from build123d import *

# Parameters (mm, degrees)
F0_R     = 50
F1_DEPTH = 10
F2_T     = -2.5
F3_W     = 4.3
F3_H     = 4.3
F4_DEPTH = 25


with BuildPart() as f1:
    # F0 (on Top) → F1 (new body)
    with BuildSketch(Plane.XY):
        with Locations((-0.804745, 0.344891)):
            Circle(F0_R)
    extrude(amount=F1_DEPTH)

    # F2
    f2_openings = [f1.faces().sort_by_distance(p)[0] for p in [
        (-0.804745, 0.344891, 10),
    ]]
    offset(amount=F2_T, openings=f2_openings)

    # F3 (on Top) → F4 (join)
    with BuildSketch(Plane.XY):
        with Locations((47.132396, -0.684507)):
            Rectangle(F3_W, F3_H)
    extrude(amount=F4_DEPTH)


solid = f1.part
Geometry check sheet. Reference: the model listing, model coordinates, mm. A direction names the side the tool comes from. Coordinates: 2 decimals unless noted, no trailing zeros. Order: outer loops, then holes, each group sorted by start corner. A loop starts at its lowest first (then second) coordinate and runs counter-clockwise, first axis right, second up. Notation, with made-up numbers: M 60.25,40.25 L 69.25,40.25 A7 ccw 69.25,52.25 Z; hole C 16,52 d6. An arc over 180 degrees is marked long. Use CSV: the item, a comma, the result in double quotes.
Item 1: Mould release check, pull along Y, two halves, no side actions. Record for faces 1 (the flat face through (47, -2.835, 15)), 2 (the flat face through (-1, 1, 2.5)), 3 (the cylindrical face through (-50.702, 3.542, 4.93)), 4 (the flat face through (47, -1, 25)): pulls with the +Y half, pulls with the -Y half, needs draft (parallel to the pull), parting line crosses it, or undercut.
Returned:
face 1,"undercut"
face 2,"undercut"
face 3,"parting line crosses it"
face 4,"needs draft"
Item 2: Gauge pin test, flat ends, axial feed: pin 1 Ø12 at (y, z) = (-22.5, 11.5) entering from +X; pin 2 Ø1 at (x, y) = (-37.5, -27) entering from +Z; pin 3 Ø6 at (y, z) = (7, 10.5) entering from +X. Record the tip position at first contact, or that the pin passes through.
Returned:
pin 1,"stops at x = 46.2"
pin 2,"stops at z = 2.5"
pin 3,"stops at x = 49.06"
Item 3: Cross-section at C-C on x = 23. Record the cut outline in (y, z), then the cut area to 3 significant figures.
Returned:
outline,"M -43.62,0 L 44.31,0 L 44.31,10 L 41.45,10 L 41.45,2.5 L -40.76,2.5 L -40.76,10 L -43.62,10 Z"
area,"263 mm2"
Item 4: Tool access check on faces 5 (the flat face through (49.282, -1, 12)), 6 (the flat face through (44.982, -1, 14)). Record the directions out of +Z, -Z, +X, -X, +Y, -Y that give a thin tool (end or side, any length) a straight path to the whole face; none if there is none.
Returned:
face 5,"+Z, -Z, +X, +Y, -Y"
face 6,"+Z"
Item 5: Thickness scan on line 1 along X through (y, z) = (-0.5, 4.5); line 2 along Z through (x, y) = (-25.5, -8.5); line 3 along X through (y, z) = (-34, 4.5). Record the ranges inside material, lowest first.
Returned:
line 1,"x = -50.8 to -48.3, 44.98 to 49.28"
line 2,"z = 0 to 2.5"
line 3,"x = -37.14 to -33.62, 32.01 to 35.53"
Item 6: Cross-section at D-D on z = 23. Record the cut outline in (x, y), then the cut area to 3 significant figures.
Returned:
outline,"M 44.98,-2.83 L 49.28,-2.83 L 49.28,1.47 L 44.98,1.47 Z"
area,"18.5 mm2"
Item 7: Cross-section at B-B on y = 41.5. Record the cut outline in (x, z).
Returned:
outline,"M -29.2,0 L 27.59,0 L 27.59,10 L 22.91,10 L 22.91,2.5 L -24.52,2.5 L -24.52,10 L -29.2,10 Z"
Item 8: Cross-section at A-A on z = 4.25. Record the cut outline in (x, y).
Returned:
outline,"M 49.09,-2.83 L 49.28,-2.83 L 49.28,1.47 L 49.18,1.47 A50 ccw long Z; hole M 44.98,-2.83 L 44.98,1.47 L 46.68,1.47 A47.5 ccw long 46.59,-2.83 Z"
